Geometry: final body of the model. Coordinates: model frame, mm. Face numbers are marked on the shaded views. A direction names the side the tool comes from. Give positions to 0.01 mm unless a question says otherwise; leave off trailing zeros. Write each loop counter-clockwise with the first axis right and the second up, starting at its lowest first coordinate (ties: lowest second). Pieces come first, ordered by that corner, then holes.
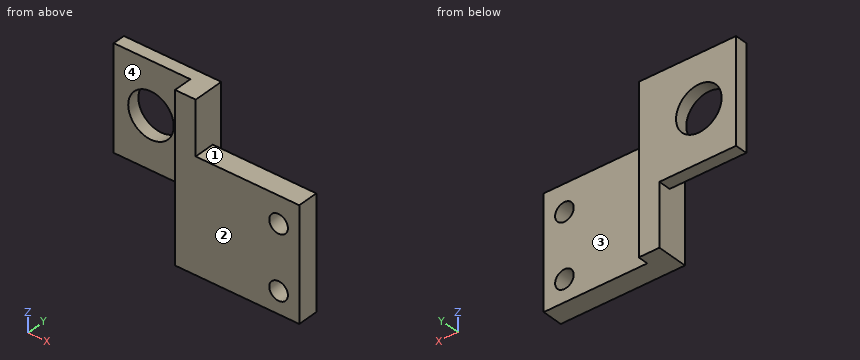
Autodesk Inventor part; units mm, degrees
ref_plane "YZ Plane" through (0, 0, 0) normal (1, 0, 0) x (0, 1, 0)
ref_plane "XZ Plane" through (0, 0, 0) normal (0, 1, 0) x (-1, 0, 0)
ref_plane "XY Plane" through (0, 0, 0) normal (0, 0, 1) x (1, 0, 0)
sketch "Sketch1" plane through (0, 0, 0) normal (0, 1, 0) x (-1, 0, 0)
  line L0 (10, 7.5) -> (10, -7.5)
  circle A0 centre (0, 0) radius 5.25
  circle A1 centre (-15.9216, -7.65) radius 2.25
  circle A2 centre (-15.8711, 7.6499) radius 2.25
  line L1 (10, 0) -> (-25.8686, 0) construction
  line L2 (10, 7.5) -> (-10.3711, 7.5)
  line L3 (-10.3711, 7.5) -> (-10.3711, 15.9691)
  line L4 (-10.3711, 15.9691) -> (-21.3711, 15.9691)
  line L5 (-21.3711, 15.9691) -> (-21.3711, -15)
  line L6 (-21.3711, -15) -> (-10.3711, -15)
  line L7 (-10.3711, -15) -> (-10.3711, -7.5)
  line L8 (-10.3711, -7.5) -> (10, -7.5)
  circle A3 centre (-15.9216, -7.65) radius 5
  circle A4 centre (-15.8711, 7.6499) radius 4.9375
  point P0 (-7.9343, 0)
  dimension "d0" = 10.5
  dimension "d2" = 10
  dimension "d3" = 15.3
  dimension "d4" = 7.65
  dimension "d5" = 4.5
  dimension "d6" = 15
  dimension "d7" = 15
  dimension "d8" = 11
  dimension "d9" = 5.5
  dimension "d10" = 10
extrude "Extrusion1" [suppressed]
sketch "Sketch2" plane through (0, 0, 0) normal (0, 0, 1) x (1, 0, 0)
  line L0 (0, 0) -> (0, 3)
  line L1 (0, 3) -> (23.5, 3)
  line L2 (23.5, 3) -> (23.5, 0.5)
  line L3 (23.5, 0.5) -> (48.5, 0.5)
  line L4 (48.5, 0.5) -> (48.5, -4.5)
  line L5 (48.5, -4.5) -> (18.5, -4.5)
  line L6 (18.5, -4.5) -> (18.5, 0)
  line L7 (18.5, 0) -> (0, 0)
  line L8 (18.5, 0) -> (18.5, 3)
  point P0 (0, 1.5)
  dimension "d13" = 3
  dimension "d14" = 5
  dimension "d15" = 25
  dimension "d16" = 23.5
  dimension "d28" = 4.5
  dimension "d29" = 5
extrude "Extrusion2" add sketch "Sketch2" against normal blind 25
sketch "Sketch3" plane through (0, 3, 0) normal (0, 1, 0) x (-1, 0, 0)
  circle A0 centre (-9, -12.5) radius 5.5
  line L0 (0, 0) -> (0, -25)
  line L1 (-23.5, 0) -> (0, 0)
  point P0 (0, -12.5)
  point P1 (0, -12.5)
  dimension "d19" = 11
  dimension "d26" = 9
  dimension "d27" = 12.5
extrude "Extrusion3" cut sketch "Sketch3" against normal blind 25
extrude "Extrusion4" add sketch "Sketch2" against normal blind 40 contours L8 L1 L2 L3 L4 L5 L6
sketch "Sketch4" plane through (23.5, 0.5, 0) normal (0, 1, 0) x (1, 0, 0)
  circle A0 centre (20, 34.7005) radius 2.25
  circle A1 centre (20, 19.4005) radius 2.25
  line L0 (0, 0) -> (0, 40)
  point P0 (-23.5, 0)
  dimension "d32" = 4.5
  dimension "d33" = 15.3
  dimension "d36" = 20
extrude "Extrusion5" cut sketch "Sketch4" against normal up to surface (5 mm away)
sketch "Sketch5" plane through (23.5, 0.5, 0) normal (0, 1, 0) x (1, 0, 0)
  line L0 (25, 0) -> (0, 0)
  line L1 (0, 0) -> (0, 40)
  line L2 (25, 0) -> (0, 0)
  line L3 (0, 0) -> (0, 12.946)
  line L4 (0, 12.946) -> (25, 12.946)
  line L5 (25, 12.946) -> (25, 0)
  point P0 (-23.5, 0)
extrude "Extrusion6" cut sketch "Sketch5" against normal blind 10
equation "\"d4\" = 0.5 * d3"
properties part number "imu2_mount" material "ABS Plastic"
Item 1: Section D-D, the plane z = -4.5. Return the cut outline in (x, y), plus the area to 3 significant figures.
Found:
outline: (0, 0) - (18.5, 0) - (18.5, -4.5) - (23.5, -4.5) - (23.5, 3) - (0, 3) - close
area: 93.0 mm2
Item 2: Line query: L1, parallel to Z at x = 43.5, y = -2.2; L2, parallel to Z at x = 9, y = 1; L3, parallel to Y at x = 15.5, z = -10. Output: solid intervals per line, ascending.
Found:
L1: z = -40 to -36.95, -32.45 to -21.65, -17.15 to -12.95
L2: z = -25 to -18, -7 to 0
L3: y = 0 to 3
Item 3: Section B-B, the plane y = 2. Return the cut outline in (x, z).
Found:
outline: (0, -25) - (18.5, -25) - (18.5, -40) - (23.5, -40) - (23.5, 0) - (0, 0) - close; hole circle Ø11 at (9, -12.5)
Item 4: Pin query (flat end, axial travel): pin 1 Ø4 at (y, z) = (0.5, -24) entering from -X; pin 2 Ø7 at (x, z) = (43.5, -34.7) entering from +Y; pin 3 Ø0.9 at (x, y) = (14, 1) entering from -Z; pin 4 Ø9 at (x, z) = (13.5, -17.5) entering from -Y. Return the tip coordinate at first contact, or that it passes through.
Found:
pin 1: stops at x = 0
pin 2: stops at y = 0.5
pin 3: stops at z = -25
pin 4: stops at y = 0
Item 5: Section C-C, the plane x = 43.5. Return the cut outline in (y, z).
Found:
outline: (-4.5, -40) - (0.5, -40) - (0.5, -36.95) - (-4.5, -36.95) - close; (-4.5, -32.45) - (0.5, -32.45) - (0.5, -21.65) - (-4.5, -21.65) - close; (-4.5, -17.15) - (0.5, -17.15) - (0.5, -12.95) - (-4.5, -12.95) - close
Item 6: Section A-A, the plane x = 9. Return the cut outline in (y, z), plus the area to 3 significant figures.
Found:
outline: (0, -25) - (3, -25) - (3, -18) - (0, -18) - close; (0, -7) - (3, -7) - (3, 0) - (0, 0) - close
area: 42.0 mm2
Item 7: Reachability of the marked faces 1, 2, 3 and 4 from +Z, -Z, +X, -X, +Y, -Y: full face, straight path, thin tool, end or side. Return the list, or none.
Found:
face 1: +Z, +X, +Y, -Y
face 2: +Z, -Z, +X, -X, -Y
face 3: +Z, -Z, +X, +Y
face 4: +Z, -Z, -X, -Y
